Here's the drawing with two shaded views (mm, measured from the low corner). I have some questions. A direction names the side the tool comes from. Give positions to 0.01 mm unless a question says otherwise; leave off trailing zeros. Write each loop counter-clockwise with the first axis right and the second up, starting at its lowest first coordinate (ties: lowest second). Pieces come first, ordered by that corner, then holes. Notation, with made-up numbers: M 87.5,3 L 93.5,3 A5 ccw 93.5,12 Z; hole C 85,-38 d10. An arc over 180 degrees is marked long. Answer as a JSON object with one key per item and string values. Group by question number.
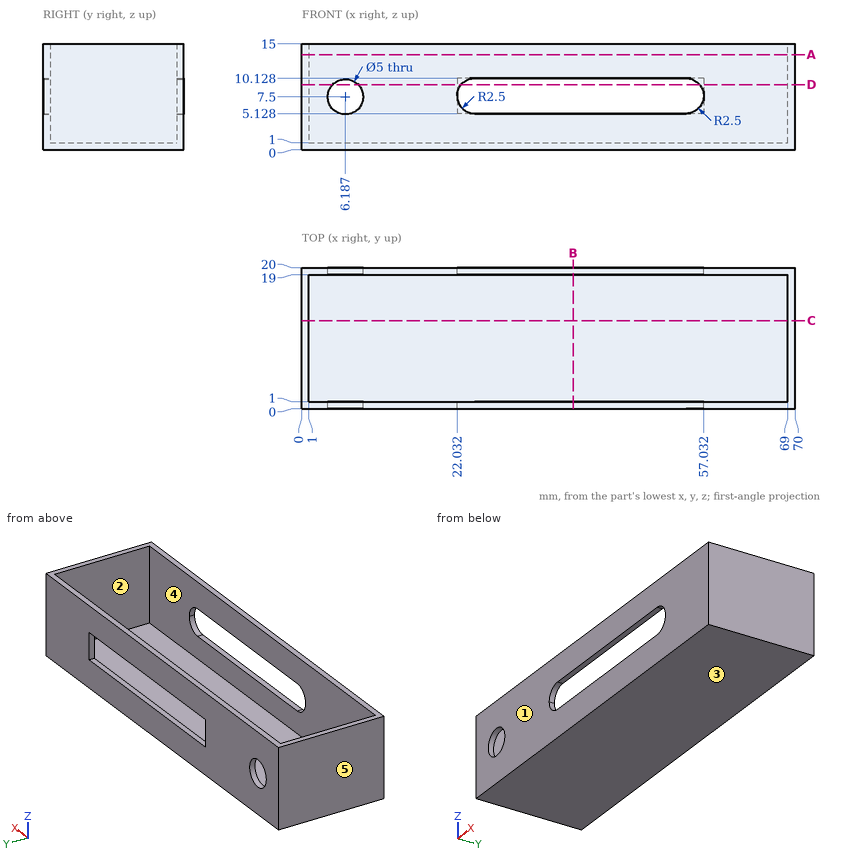
1) If we section it at B-B, the plane x = 38.5: List the corners of the cut face in (y, z) for me.
2) If we section it at D-D, the plane z = 9.25: List the corners of the cut face in (x, y) for me (1 decimal).
3) If we section it at A-A, the plane z = 13.5: List the corners of the cut face in (x, y) for me.
4) Please list where these lines run through material, in increasing order: line 1 along Y through (x, z) = (67, 4.5); line 2 along X through (y, z) = (5, 12.5); line 3 along X through (y, z) = (19.25, 6.5) (1 decimal). Write a range as from..to.
5) I'm going to push a flat-ended pin straight in: pin 1 (8 mm diameter, centred on x = 55.5, y = 10.5, fed in from +Z). Where does the tip first touch, or does it pass through?
6) If we section it at C-C, the plane y = 12.5: List the corners of the cut face in (x, z) for me.
7) For the marked faces 1 and 2, which set-ups out of +Z, -Z, +X, -X, +Y, -Y let a thin tool reach every point of the face, with its end or its side?
8) We'd pull the mould along X, two halves only. Please class the marked faces 3, 4 and 5: released by +X, released by -X, zero draft, split by the parting line, or undercut.
Taken from the geometry:
{
 "1": {"outline": "M 0,0 L 20,0 L 20,5.13 L 19,5.13 L 19,1 L 1,1 L 1,5.13 L 0,5.13 Z; M 0,10.13 L 1,10.13 L 1,15 L 0,15 Z; M 19,10.13 L 20,10.13 L 20,15 L 19,15 Z"},
 "2": {"outline": "M 0,0 L 4.4,0 L 4.4,1 L 1,1 L 1,19 L 4.4,19 L 4.4,20 L 0,20 Z; M 8,0 L 22.6,0 L 22.6,1 L 8,1 Z; M 8,19 L 22,19 L 22,20 L 8,20 Z; M 56.4,0 L 70,0 L 70,20 L 57,20 L 57,19 L 69,19 L 69,1 L 56.4,1 Z"},
 "3": {"outline": "M 0,0 L 70,0 L 70,20 L 0,20 Z; hole M 1,1 L 69,1 L 69,19 L 1,19 Z"},
 "4": {"line 1": "0..1, 19..20", "line 2": "0..1, 69..70", "line 3": "0..3.9, 8.5..22, 57..70"},
 "5": {"pin 1": "z = 1"},
 "6": {"outline": "M 0,0 L 70,0 L 70,15 L 69,15 L 69,1 L 1,1 L 1,15 L 0,15 Z"},
 "7": {"face 1": "+Z, -Z, +X, -X, -Y", "face 2": "+Z"},
 "8": {"face 3": "zero draft", "face 4": "undercut", "face 5": "released by -X"}
}
